Verification items for the finished model (mm, model axes). A direction names the side the tool comes from. Coordinates: 2 decimals unless noted, no trailing zeros. Write each loop counter-clockwise with the first axis right and the second up, starting at its lowest first coordinate (ties: lowest second). Pieces come first, ordered by that corner, then holes. Notation, with made-up numbers: (76, 45) -> (108, 45) arc R21 cw to (108, 71) -> close; hole circle Ø3 at (-28.5, 5). An arc over 180 degrees is marked (long way). Answer in a Markdown table with one row per item.
```python
from build123d import *

# Parameters (mm, degrees)
F0_R     = 3.5
F1_DEPTH = 8.89
F2_DEPTH = 38.1
F3_DEPTH = 13.97


with BuildPart() as f1:
    # F0 (on Front) → F1 (new body)
    with BuildSketch(Plane.XZ):
        Polygon((12.192, -3.96875), (12.192, 3.96875), (3.96875, 3.96875), (3.96875, 12.192), (-3.96875, 12.192), (-3.96875, 3.96875), (-12.192, 3.96875), (-12.192, -3.96875), (-3.96875, -3.96875), (-3.96875, -12.192), (3.96875, -12.192), (3.96875, -3.96875), align=None)
        Circle(F0_R, mode=Mode.SUBTRACT)
    extrude(amount=F1_DEPTH)

    # F0 (on Front) → F2 (join)
    with BuildSketch(Plane.XZ):
        Circle(F0_R)
    extrude(amount=F2_DEPTH)

    # F0 (on Front) → F3 (join)
    with BuildSketch(Plane.XZ):
        Circle(F0_R)
    extrude(amount=-F3_DEPTH)


solid = f1.part
```
1. Sectioned sample at B-B, the plane x = 0. Record the cut outline in (y, z).
Findings below:
| item | result |
|---|---|
| outline | (-38.1, -3.5) -> (-8.89, -3.5) -> (-8.89, -12.19) -> (0, -12.19) -> (0, -3.5) -> (13.97, -3.5) -> (13.97, 3.5) -> (0, 3.5) -> (0, 12.19) -> (-8.89, 12.19) -> (-8.89, 3.5) -> (-38.1, 3.5) -> close |
2. Go/stop test with flat-tipped pins: pin 1 (4 mm diameter, centred on y = -6, z = 9.5, fed in from +X); pin 2 (2.5 mm diameter, centred on x = -9.5, y = -3.5, fed in from +Z); pin 3 (4 mm diameter, centred on x = 1.5, z = -8.5, fed in from -Y). Record where each tip stops, or that it passes through.
Findings below:
| item | result |
|---|---|
| pin 1 | stops at x = 3.97 |
| pin 2 | stops at z = 3.97 |
| pin 3 | stops at y = -8.89 |
3. Sectioned sample at D-D, the plane z = 5.5. Record the cut outline in (x, y).
Findings below:
| item | result |
|---|---|
| outline | (-3.97, -8.89) -> (3.97, -8.89) -> (3.97, 0) -> (-3.97, 0) -> close |
4. Sectioned sample at C-C, the plane y = -20. Record the cut outline in (x, z), and give its area (3 significant figures).
Findings below:
| item | result |
|---|---|
| outline | circle Ø7 at (0, 0) |
| area | 38.5 mm² |
5. Sectioned sample at A-A, the plane z = 0. Record the cut outline in (x, y), and give its area (3 significant figures).
Findings below:
| item | result |
|---|---|
| outline | (-12.19, -8.89) -> (-3.5, -8.89) -> (-3.5, -38.1) -> (3.5, -38.1) -> (3.5, -8.89) -> (12.19, -8.89) -> (12.19, 0) -> (3.5, 0) -> (3.5, 13.97) -> (-3.5, 13.97) -> (-3.5, 0) -> (-12.19, 0) -> close |
| area | 519 mm² |
6. Material ranges on probe 1 along Y at (x, z) = (7.5, 3.25); probe 2 along X at (y, z) = (-1, -7), recorded low to high. Write a range as from..to.
Findings below:
| item | result |
|---|---|
| probe 1 | y = -8.89..0 |
| probe 2 | x = -3.97..3.97 |
7. Access from +Z, -Z, +X, -X, +Y, -Y to the whole of each face (thin tool, end or side, straight path). Record for faces 1 (the face through (8, -4, -3.969)), 2 (the face through (3.969, -4, 8)), 3 (the face through (3.233, -23.291, -1.341)), 4 (the face through (-8, -4, -3.969)), 5 (the face through (-8, -4, 3.969)).
Findings below:
| item | result |
|---|---|
| face 1 | -Z, +X, +Y, -Y |
| face 2 | +Z, +X, +Y, -Y |
| face 3 | -Y |
| face 4 | -Z, -X, +Y, -Y |
| face 5 | +Z, -X, +Y, -Y |
